from build123d import *

# Parameters (mm, degrees)
F0_R     = 4
F0_R_2   = 2.75
F1_DEPTH = 2
F2_DEPTH = 13
F4_DEPTH = 5
F8_R     = 1
F9_DEPTH = 45


with BuildPart() as f1:
    # F0 (on Top) → F1 (new body)
    with BuildSketch(Plane.XY):
        Circle(F0_R)
        Circle(F0_R_2, mode=Mode.SUBTRACT)
        Circle(F0_R_2)
    extrude(amount=F1_DEPTH)

    # F0 (on Top) → F2 (join)
    with BuildSketch(Plane.XY):
        Circle(F0_R_2)
    extrude(amount=-F2_DEPTH)

    # F3 (on face) → F4 (join)
    with BuildSketch(Plane(origin=(0, 0, -13), x_dir=(1, 0, 0), z_dir=(0, 0, -1))):
        Polygon((1.0625, -1.840304), (2.125, 0), (1.0625, 1.840304), (-1.0625, 1.840304), (-2.125, 0), (-1.0625, -1.840304), align=None)
    extrude(amount=F4_DEPTH)

    # F8 (on offset) → F9 (cut)
    with BuildSketch(Plane.XZ.offset(25)):
        with Locations((0, -6)):
            Circle(F8_R)
    extrude(amount=-F9_DEPTH, mode=Mode.SUBTRACT)


solid = f1.part
Build history of the part. All positions in model axes, mm. A direction names the side the tool comes from. Round coordinates to 2 decimals unless told otherwise and drop trailing zeros. Loops run counter-clockwise (first coordinate to the right, second up) from the corner with the lowest first, then second, coordinate; pieces in that order, holes last. Notation, with made-up numbers: (24.5, -16.75) -> (62.5, -16.75) arc R21 cw to (62.5, 15.25) -> close; hole circle Ø8 at (76, 47). An arc over 180 degrees is marked (long way). One line per item, written item: value. Start each with the question number.
Q1. Probe line 1 along Z through (x, y) = (0, 0.45); line 2 along Z through (x, y) = (2.75, -1.5); line 3 along Y through (x, z) = (0, -8.75). List the from-to ranges inside material, lowest first.
Q2. Two-plate mould, pull along Z, no slides. Class faces 1 (the face through (0, 0, -5)), 2 (the face through (2, 1, -13)), 3 (the face through (1.6, -0.91, -15.46)): released by +Z, released by -Z, zero draft, split by the parting line, or undercut.
Q3. Cut at D-D on z = -3.75. List the corners of the cut face in (x, y).
Q4. Cut at C-C on y = -1.25. List the corners of the cut face in (x, z), plus the area to 3 significant figures.
Q5. Drop flat-ended pins along their axis: pin 1 Ø1.7 at (x, z) = (0, -15) entering from +Y; pin 2 Ø1.5 at (y, z) = (-1.5, -10.5) entering from +X; pin 3 Ø1.7 at (x, z) = (0, -14.5) entering from -Y. Give the stop position or say it passes through.
Q6. 3-axis set-ups, long thin cutter, end or side, ignore diameter. For faces 4 (the face through (0, -1.84, -15)), 5 (the face through (2.54, -1.05, -6.41)), 6 (the face through (0, 1.84, -15)), 7 (the face through (-1.59, -0.93, -15.46)), 8 (the face through (-1.6, 0.91, -15.46)): which of +Z, -Z, +X, -X, +Y, -Y reach the whole face in a straight line?
Q7. Cut at B-B on z = -6. List the corners of the cut face in (x, y), plus the area to 3 significant figures.
Q8. Cut at A-A on x = 0. List the corners of the cut face in (y, z).
Computed:
1. line 1: -18 to -7, -5 to 2
1. line 2: 0 to 2
1. line 3: -2.75 to 2.75
2. face 1: undercut
2. face 2: released by -Z
2. face 3: zero draft
3. outline: circle Ø5.5 at (0, 0)
4. outline: (-3.8, 0) -> (-2.45, 0) -> (-2.45, -13) -> (-1.4, -13) -> (-1.4, -18) -> (1.4, -18) -> (1.4, -13) -> (2.45, -13) -> (2.45, 0) -> (3.8, 0) -> (3.8, 2) -> (-3.8, 2) -> close; hole circle Ø2 at (0, -6)
4. area: 89.8 mm²
5. pin 1: y = 1.84
5. pin 2: x = 2.65
5. pin 3: y = -1.84
6. face 4: -Z, +X, -X, -Y
6. face 5: -Z
6. face 6: -Z, +X, -X, +Y
6. face 7: -Z, -X, -Y
6. face 8: -Z, -X, +Y
7. outline: (-1, -2.56) -> (-1, 2.56) arc R2.75 ccw to start; (1, -2.56) arc R2.75 ccw to (1, 2.56) -> close
7. area: 13.0 mm²
8. outline: (-4, 0) -> (-2.75, 0) -> (-2.75, -5) -> (2.75, -5) -> (2.75, 0) -> (4, 0) -> (4, 2) -> (-4, 2) -> close; (-2.75, -13) -> (-1.84, -13) -> (-1.84, -18) -> (1.84, -18) -> (1.84, -13) -> (2.75, -13) -> (2.75, -7) -> (-2.75, -7) -> close
